from build123d import *

# Parameters (mm, degrees)
SKETCH1_W           = 40
SKETCH1_H           = 5
BOSS_EXTRUDE1_DEPTH = 20
SKETCH2_R           = 28.5
CUT_EXTRUDE1_DEPTH  = 21
CUT_EXTRUDE1_TAPER  = -7
SKETCH3_R           = 1.35
CUT_EXTRUDE2_DEPTH  = 6.0000001


with BuildPart() as part:
    # Sketch1 → Boss-Extrude1 (new body)
    with BuildSketch(Plane.XY):
        with Locations((-20, -2.5)):
            Rectangle(SKETCH1_W, SKETCH1_H)
        Polygon((-40, -5), (-40, 0), (-110, 0), (-110, -50), (-40, -50), align=None)
    extrude(amount=BOSS_EXTRUDE1_DEPTH)

    # Sketch2 → Cut-Extrude1 (cut, through all)
    with BuildSketch(Plane.XY.offset(20)):
        with Locations((-75, 0)):
            Circle(SKETCH2_R)
    extrude(amount=-CUT_EXTRUDE1_DEPTH, taper=CUT_EXTRUDE1_TAPER, mode=Mode.SUBTRACT)

    # Sketch3 → Cut-Extrude2 (cut, through all)
    with BuildSketch(Plane.XZ.offset(5)):
        with Locations((-23, 5)):
            Circle(SKETCH3_R)
        with Locations((-11, 5)):
            Circle(SKETCH3_R)
    extrude(amount=-CUT_EXTRUDE2_DEPTH, mode=Mode.SUBTRACT)


solid = part.part
Read the model definition and answer for the solid it produces. Units are mm, in the model's axes. A direction names the side the tool comes from. Coordinates: 2 decimals unless noted, no trailing zeros. Order: outer loops, then holes, each group sorted by start corner. A loop starts at its lowest first (then second) coordinate and runs counter-clockwise, first axis right, second up. Notation, with made-up numbers: M 35.5,27 L 41.5,27 A17 ccw 41.5,46 Z; hole C 5.25,40 d3. An arc over 180 degrees is marked long. Put each result on its own line as item: value. Start each with the question number.
Item 1: Section A-A, the plane x = -23 is taken. Determine the outline of the cut face in (y, z).
Item 2: Consider probe 1 along Z at (x, y) = (-11, -2.9); probe 2 along Y at (x, z) = (-15, 1.75); probe 3 along X at (y, z) = (-45, 11). Determine where each line is inside the solid, lowest interval first. Write a range as [from, to].
Item 3: For faces 4 (the face through (-75.648, -29.465, 12.082)), 5 (the face through (-20, -5, 10)), determine the directions among +Z, -Z, +X, -X, +Y, -Y from which every point of the face is accessible in a straight line to the end or side of a thin tool.
Item 4: The mould has two halves that part along Z. Classify faces 1 (the face through (-21.712, -2.535, 5.406)), 2 (the face through (-40, -28, 10)), 3 (the face through (-68, -30, 20)): +Z half, -Z half, draft (parallel to the pull), parting line (faces both ways), or undercut.
Item 5: Section C-C, the plane z = 15.5 is taken. Determine the outline of the cut face in (x, y), plus the area to 3 significant figures.
Item 6: Section D-D, the plane y = -47 is taken. Determine the outline of the cut face in (x, z).
Item 7: Section B-B, the plane z = 5 is taken. Determine the outline of the cut face in (x, y).
Item 8: Given pin 1 Ø6 at (y, z) = (-19, 15) entering from +X; pin 2 Ø8 at (x, z) = (-55, 3) entering from +Y, each flat-ended and moving along its own axis, determine where each tip first touches the part or whether it passes through.
Computed:
1. outline: M -5,0 L 0,0 L 0,3.65 L -5,3.65 Z; M -5,6.35 L 0,6.35 L 0,20 L -5,20 Z
2. probe 1: z = [0, 3.65], [6.35, 20]
2. probe 2: y = [-5, 0]
2. probe 3: x = [-110, -40]
3. face 4: -Z, +Y
3. face 5: +Z, -Z, +X, -Y
4. face 1: undercut
4. face 2: draft
4. face 3: +Z half
5. outline: M -110,-50 L -40,-50 L -40,-5 L 0,-5 L 0,0 L -45.95,0 A29.05 cw -104.05,0 L -110,0 Z
5. area: 2,370 mm2
6. outline: M -110,0 L -40,0 L -40,20 L -110,20 Z
7. outline: M -110,-50 L -40,-50 L -40,-5 L -24.35,-5 L -24.35,0 L -44.66,0 A30.34 cw -105.34,0 L -110,0 Z; M -21.65,-5 L -12.35,-5 L -12.35,0 L -21.65,0 Z; M -9.65,-5 L 0,-5 L 0,0 L -9.65,0 Z
8. pin 1: stops at x = -40
8. pin 2: stops at y = -18.9
